Could you check a few things on this model? Use its own coordinates, in mm. A direction names the side the tool comes from. Give positions to 0.01 mm unless a question says otherwise; leave off trailing zeros. Write each loop counter-clockwise with the first axis right and the second up, starting at its lowest first coordinate (ties: lowest second). Pieces come first, ordered by that corner, then holes. Notation, with made-up numbers: (25, 60) -> (81, 60) arc R22 ccw to (81, 82) -> close; hole circle Ø5 at (51.25, 3.5). An arc over 180 degrees is marked (long way). One line per question, with ' | ' between items.
from build123d import *

# Parameters (mm, degrees)
SKETCH1_W           = 90
SKETCH1_H           = 90
BOSS_EXTRUDE1_DEPTH = 2000
SKETCH2_W           = 90
SKETCH2_H           = 90
CUT_EXTRUDE1_DEPTH  = 45
SKETCH3_W           = 90
SKETCH3_H           = 90
CUT_EXTRUDE2_DEPTH  = 45


with BuildPart() as part:
    # Sketch1 → Boss-Extrude1 (new body)
    with BuildSketch(Plane(origin=(0, 0, 0), x_dir=(0, 0, -1), z_dir=(1, 0, 0))):
        with Locations((45, 45)):
            Rectangle(SKETCH1_W, SKETCH1_H)
    extrude(amount=BOSS_EXTRUDE1_DEPTH)

    # Sketch2 → Cut-Extrude1 (cut)
    with BuildSketch(Plane(origin=(0, 90, 0), x_dir=(1, 0, 0), z_dir=(0, 1, 0))):
        with Locations((45, 45)):
            Rectangle(SKETCH2_W, SKETCH2_H)
        with Locations((1955, 45)):
            Rectangle(SKETCH2_W, SKETCH2_H)
    extrude(amount=-CUT_EXTRUDE1_DEPTH, mode=Mode.SUBTRACT)

    # Sketch3 → Cut-Extrude2 (cut)
    with BuildSketch(Plane(origin=(0, 0, -90), x_dir=(-1, 0, 0), z_dir=(0, 0, -1))):
        with Locations((-1555, 45)):
            Rectangle(SKETCH3_W, SKETCH3_H)
        with Locations((-445, 45)):
            Rectangle(SKETCH3_W, SKETCH3_H)
    extrude(amount=-CUT_EXTRUDE2_DEPTH, mode=Mode.SUBTRACT)


solid = part.part
Q1. If we mould it in two halves opening along X, with no side actions, what happens to faces 5 (the flat face through (1910, 68, -44)), 6 (the flat face through (987, 90, -44)), 7 (the flat face through (1556, 46, -45))? For each: +X half, -X half, draft (parallel to the pull), parting line (faces both ways), or undercut.
Answer below:
face 5: +X half | face 6: draft | face 7: undercut
Q2. Will these pins go through, and if not, where does the flat tip stop? pin 1 (13.5 mm diameter, centred on y = 55.5, z = -62.5, fed in from -X); pin 2 (22.5 mm diameter, centred on y = 63.5, z = -43, fed in from +X).
Answer below:
pin 1: stops at x = 90 | pin 2: stops at x = 1910
Q3. Imagine slicing it at A-A on z = -65. Please give me the cut outline in (x, y).
Answer below:
outline: (0, 0) -> (400, 0) -> (400, 90) -> (90, 90) -> (90, 45) -> (0, 45) -> close; (490, 0) -> (1510, 0) -> (1510, 90) -> (490, 90) -> close; (1600, 0) -> (2000, 0) -> (2000, 45) -> (1910, 45) -> (1910, 90) -> (1600, 90) -> close
Q4. If I drill on line 1 along X through (y, z) = (35, -49); line 2 along X through (y, z) = (50, -70); line 3 along X through (y, z) = (60.5, -26), over which ranges is the centre line in solid material (lowest first)?
Answer below:
line 1: x = 0 to 400, 490 to 1510, 1600 to 2000 | line 2: x = 90 to 400, 490 to 1510, 1600 to 1910 | line 3: x = 90 to 1910
Q5. Imagine slicing it at C-C on x = 1577. Please give me the cut outline in (y, z).
Answer below:
outline: (0, -45) -> (90, -45) -> (90, 0) -> (0, 0) -> close
Q6. Imagine slicing it at B-B on y = 20.5. Please give me the cut outline in (x, z), and give its area (3 significant figures).
Answer below:
outline: (0, -90) -> (400, -90) -> (400, -45) -> (490, -45) -> (490, -90) -> (1510, -90) -> (1510, -45) -> (1600, -45) -> (1600, -90) -> (2000, -90) -> (2000, 0) -> (0, 0) -> close | area: 172,000 mm^2
Q7. On a 3-axis mill with a long thin cutter (end or side, diameter ignored), from which of +Z, -Z, +X, -X, +Y, -Y can I reach the whole of each face in a straight line? I mean faces 1 (the flat face through (44, 45, -46)), 2 (the flat face through (1510, 44, -68)), 3 (the flat face through (2000, 23, -44)), 4 (the flat face through (1954, 45, -46)). Say none if no direction works.
Answer below:
face 1: +Z, -Z, -X, +Y | face 2: -Z, +Y, -Y | face 3: +Z, -Z, +X, +Y, -Y | face 4: +Z, -Z, +X, +Y
